```python
from build123d import *

# Parameters (mm, degrees)
SKETCH1_W                = 25.4
SKETCH1_H                = 25.4
SKETCH1_W_2              = 23
SKETCH1_H_2              = 23
BOSS_EXTRUDE1_DEPTH      = 499.2
SKETCH3_W                = 25.4
SKETCH3_H                = 5
BOSS_EXTRUDE2_DEPTH      = 1
BOSS_EXTRUDE2_DEPTH_BACK = 26.4


with BuildPart() as part:
    # Sketch1 → Boss-Extrude1 (new body)
    with BuildSketch(Plane(origin=(0, 0, 0), x_dir=(1, 0, 0), z_dir=(0, 1, 0))):
        with Locations((12.7, 12.7)):
            Rectangle(SKETCH1_W, SKETCH1_H)
        with Locations((12.7, 12.7)):
            Rectangle(SKETCH1_W_2, SKETCH1_H_2, mode=Mode.SUBTRACT)
    extrude(amount=BOSS_EXTRUDE1_DEPTH)

    # Sketch3 → Boss-Extrude2 (add, two sides)
    with BuildSketch(Plane(origin=(0, 0, -25.4), x_dir=(-1, 0, 0), z_dir=(0, 0, -1))) as boss_extrude2_sk:
        with Locations((-12.7, 104.2)):
            Rectangle(SKETCH3_W, SKETCH3_H)
        with Locations((-12.7, 134.6)):
            Rectangle(SKETCH3_W, SKETCH3_H)
        with Locations((-12.7, 395)):
            Rectangle(SKETCH3_W, SKETCH3_H)
        with Locations((-12.7, 364.6)):
            Rectangle(SKETCH3_W, SKETCH3_H)
    extrude(amount=BOSS_EXTRUDE2_DEPTH)
    extrude(boss_extrude2_sk.sketch, amount=-BOSS_EXTRUDE2_DEPTH_BACK)


solid = part.part
```
Input: part model. Units: mm. Frame: model coordinates. A direction names the side the tool comes from. Coordinates: 2 decimals unless noted, no trailing zeros. Write each loop counter-clockwise with the first axis right and the second up, starting at its lowest first coordinate (ties: lowest second). Pieces come first, ordered by that corner, then holes. Notation, with made-up numbers: M -7.5,32 L 18.5,32 A22 cw 18.5,54 Z; hole C 52,23.25 d7. An arc over 180 degrees is marked long. Use one line per item in the form item = value.
Q1. Section A-A (y = 426). Return loops of the section in (x, z).
Answer below:
outline = M 0,-25.4 L 25.4,-25.4 L 25.4,0 L 0,0 Z; hole M 1.2,-24.2 L 24.2,-24.2 L 24.2,-1.2 L 1.2,-1.2 Z
Q2. Section B-B (z = -11.75). Return loops of the section in (x, y).
Answer below:
outline = M 0,0 L 1.2,0 L 1.2,101.7 L 24.2,101.7 L 24.2,0 L 25.4,0 L 25.4,499.2 L 24.2,499.2 L 24.2,397.5 L 1.2,397.5 L 1.2,499.2 L 0,499.2 Z; hole M 1.2,106.7 L 24.2,106.7 L 24.2,132.1 L 1.2,132.1 Z; hole M 1.2,137.1 L 24.2,137.1 L 24.2,362.1 L 1.2,362.1 Z; hole M 1.2,367.1 L 24.2,367.1 L 24.2,392.5 L 1.2,392.5 Z
Q3. Draft query along X for faces 5 (the face through (13, 119, 0)), 6 (the face through (13, 397.5, -13)), 7 (the face through (25.4, 246, -13)). Return one class per face: released by +X, released by -X, zero draft, split by the parting line, or undercut.
Answer below:
face_5 = zero draft
face_6 = undercut
face_7 = released by +X
Q4. Section C-C (x = 18). Count the separate pieces of the cut face and the enclosed holes in it, plus the area to 3 significant figures.
Answer below:
separate_pieces = 1
enclosed_holes = 3
area = 1,700 mm²
Q5. Set-up query: faces 1 (the face through (13, 367.1, -13)), 2 (the face through (13, 101.7, -13)), 3 (the face through (13, 380, 0)), 4 (the face through (1.2, 448, -13)). Return all of +Z, -Z, +X, -X, +Y, -Y with unobstructed straight access to the full face (end or side cutting, diameter ignored); none if empty.
Answer below:
face_1 = none
face_2 = -Y
face_3 = +Z, +X, -X
face_4 = +Y
Q6. Material intervals for probe 1 along Y at (x, z) = (18, -20.75); probe 2 along Z at (x, y) = (1.5, 50); probe 3 along X at (y, z) = (210, -13.25), sorted ascending. Write a range as from..to.
Answer below:
probe_1 = 101.7..106.7, 132.1..137.1, 362.1..367.1, 392.5..397.5
probe_2 = -25.4..-24.2, -1.2..0
probe_3 = 0..1.2, 24.2..25.4
Q7. First-contact query: pin 1 (0.8 mm diameter, centred on x = 6.5, z = 0.5, fed in from -Y); pin 2 (11.5 mm diameter, centred on x = 13.5, z = -13, fed in from +Y); pin 3 (2 mm diameter, centred on x = 22, y = 411, fed in from -Z). Flat tips, straight axial feed; report the tip coordinate or a pass-through.
Answer below:
pin_1 = 101.7
pin_2 = 397.5
pin_3 = -25.4
